Here's how the part is built. I have some questions about the finished solid (model axes, mm). A direction names the side the tool comes from. Coordinates: 2 decimals unless noted, no trailing zeros.
Item 1: I want a section at B-B (x = 0). Count the separate pieces of the cut face and the enclosed holes in it, and give its area (3 significant figures).
Item 2: For faces 4 (the face through (-6.35, 5, 18)), 5 (the face through (-1.03, 1.58, -25.38)), 6 (the face through (-3, 3.969, -6)), 7 (the face through (-2.75, -3.19, -12.4)), which set-ups out of +Z, -Z, +X, -X, +Y, -Y let a thin tool reach every point of the face, with its end or its side?
Item 3: If we mould it in two halves opening along X, with no side actions, what happens to faces 1 (the face through (18.44, -0.03, 8.9)), 2 (the face through (-6.883, -0.011, -30.995)), 3 (the face through (-14.3, -0.794, 21.3))? For each: pulls with the +X half, pulls with the -X half, needs draft (parallel to the pull), parting line crosses it, or undercut.
Item 4: I'm going to push flat-ended pins straight in: P1, Ø12, axis at x = 1.5, z = 1.5, coming from the +Y side; P2, Ø2, axis at x = 7.5, z = 10, coming from the +Y side; P3, Ø3, axis at x = 1.5, z = 22.5, coming from the -Y side; P4, Ø5.5, axis at y = 4, z = 18, coming from the -X side. Where does each tip first touch, or does it pass through?
Item 5: Please list where these lines run through material, in increasing order: line 1 (Y direction, x = 0, z = 16) (1 decimal); line 2 (X direction, y = 15.5, z = 0).
from build123d import *

# Parameters (mm, degrees)
SKETCH3_W           = 6.35
SKETCH3_H           = 38.1
EXTRUDE_THIN1_START = -30.48
EXTRUDE_THIN1_DEPTH = 30.48
HOLE1_D             = 9.525
HOLE1_DEPTH         = 38.1
HOLE2_D             = 9.525
HOLE3_D             = 3.175


with BuildPart() as part:
    # Sketch1 → Revolve1 (revolve)
    with BuildSketch(Plane.XY):
        Polygon((0, 20.6375), (6.35, 20.6375), (6.35, 3.96875), (12.7, 3.96875), (12.7, 2.38125), (25.4, 2.38125), (25.4, 0.79375), (31.75, 0.79375), (31.75, -0.79375), (25.4, -0.79375), (25.4, -2.38125), (12.7, -2.38125), (12.7, -3.96875), (6.35, -3.96875), (0, -3.96875), align=None)
    revolve(axis=Axis((0, 20.6375, 0), (0, -1, 0)))

    # Sketch3 → Revolve2 (revolve)
    with BuildSketch(Plane(origin=(0, 7.9375, 0), x_dir=(1, 0, 0), z_dir=(0, 1, 0))):
        with Locations((3.175, -19.05)):
            Rectangle(SKETCH3_W, SKETCH3_H)
    revolve(axis=Axis((0, 7.9375, 0), (0, 0, 1)))

    # Sketch4 → Extrude-Thin1 (add)
    with BuildSketch(Plane.XY.offset(30.48).offset(EXTRUDE_THIN1_START)):
        Polygon((6.35, 7.9375), (6.35, 0.79375), (-6.35, 0.79375), (-6.35, 7.9375), (-3.81, 7.9375), (-3.81, 3.33375), (3.81, 3.33375), (3.81, 7.9375), align=None)
    extrude(amount=EXTRUDE_THIN1_DEPTH)

    # Hole1
    with Locations(Plane.XY.offset(38.1)):
        with Locations((0, 7.9375)):
            Hole(HOLE1_D / 2, depth=HOLE1_DEPTH)

    # Hole2 (through all)
    with Locations(Plane(origin=(0, 20.6375, 0), x_dir=(1, 0, 0), z_dir=(0, 1, 0))):
        with Locations((0, 0)):
            Hole(HOLE2_D / 2)

    # Hole3 (through all)
    with Locations(Plane(origin=(0, 2.38125, 0), x_dir=(1, 0, 0), z_dir=(0, 1, 0))):
        with Locations((0, 19.939), (17.267680526, -9.9695), (-17.267680526, -9.9695)):
            Hole(HOLE3_D / 2)


solid = part.part
Answer:
1. separate pieces: 4
1. enclosed holes: 0
1. area: 369 mm2
2. face 4: +Z, -X, +Y
2. face 5: +Y
2. face 6: -Z, +Y
2. face 7: -Y
3. face 1: undercut
3. face 2: parting line crosses it
3. face 3: needs draft
4. P1: stops at y = 20.64
4. P2: stops at y = 3.97
4. P3: stops at y = -2.38
4. P4: stops at x = -19.91
5. line 1: y = -2.4 to 3.2, 12.7 to 14.3
5. line 2: x = -6.35 to -4.76, 4.76 to 6.35
